Here's how the part is built. I have some questions about the finished solid (model axes, mm). Face numbers are marked on the shaded views. A direction names the side the tool comes from. Round coordinates to 2 decimals unless told otherwise and drop trailing zeros. Loops run counter-clockwise (first coordinate to the right, second up) from the corner with the lowest first, then second, coordinate; pieces in that order, holes last. Notation, with made-up numbers: M 55.25,34.5 L 94.25,34.5 A19 cw 94.25,49.5 Z; hole C 65,82.5 d3. An arc over 180 degrees is marked long. Use a Markdown table: item, result.
```python
from build123d import *

# Parameters (mm, degrees)
F1_DEPTH = 25.4
F0_R     = 19.05
F2_DEPTH = 38.1
F0_R_2   = 6.35
F3_DEPTH = 31.75


with BuildPart() as f1:
    # F0 (on Top) → F1 (new body)
    with BuildSketch(Plane.XY):
        with BuildLine():
            ThreePointArc((256.328097, 0.145331), (242.358097, 12.781672), (256.328097, 25.418012))
            Line((256.328097, 25.418012), (130.598097, 38.054353))
            ThreePointArc((130.598097, 38.054353), (146.895241, 29.82051), (153.458097, 12.781672))
            ThreePointArc((153.458097, 12.781672), (146.895241, -4.257166), (130.598097, -12.491009))
            Line((130.598097, -12.491009), (256.328097, 0.145331))
        make_face()
        with BuildLine():
            ThreePointArc((166.158097, 6.431672), (159.808097, 12.781672), (166.158097, 19.131672))
            Line((166.158097, 19.131672), (216.958097, 19.131672))
            ThreePointArc((216.958097, 19.131672), (223.308097, 12.781672), (216.958097, 6.431672))
            Line((216.958097, 6.431672), (166.158097, 6.431672))
        make_face(mode=Mode.SUBTRACT)
    extrude(amount=F1_DEPTH)

    # F0 (on Top) → F2 (join)
    with BuildSketch(Plane.XY):
        with BuildLine():
            ThreePointArc((153.458097, 12.781672), (146.895241, 29.82051), (130.598097, 38.054353))
            ThreePointArc((130.598097, 38.054353), (102.658097, 12.781672), (130.598097, -12.491009))
            ThreePointArc((130.598097, -12.491009), (146.895241, -4.257166), (153.458097, 12.781672))
        make_face()
        with Locations((128.058097, 12.781672)):
            Circle(F0_R, mode=Mode.SUBTRACT)
    extrude(amount=F2_DEPTH)

    # F0 (on Top) → F3 (join)
    with BuildSketch(Plane.XY):
        with BuildLine():
            ThreePointArc((256.328097, 0.145331), (264.476669, 4.262253), (267.758097, 12.781672))
            ThreePointArc((267.758097, 12.781672), (264.476669, 21.301091), (256.328097, 25.418012))
            ThreePointArc((256.328097, 25.418012), (242.358097, 12.781672), (256.328097, 0.145331))
        make_face()
        with Locations((255.058097, 12.781672)):
            Circle(F0_R_2, mode=Mode.SUBTRACT)
    extrude(amount=F3_DEPTH)


solid = f1.part
```
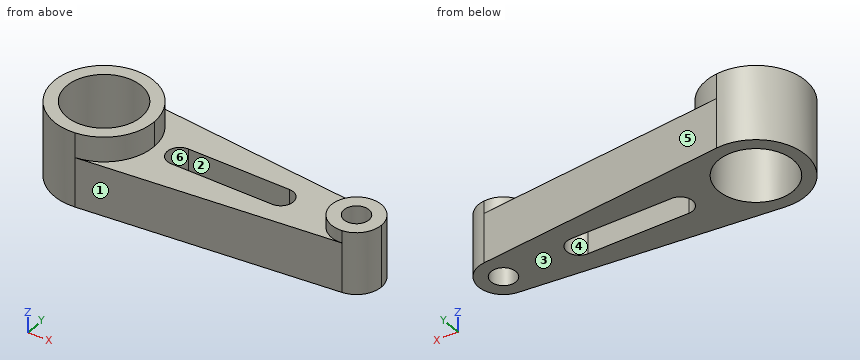
Q1. For the marked faces 1 and 2, which set-ups out of +Z, -Z, +X, -X, +Y, -Y let a thin tool reach every point of the face, with its end or its side?
Return value:
| item | result |
|---|---|
| face 1 | +Z, -Z, +X, -Y |
| face 2 | +Z, -Z |
Q2. Imagine slicing it at D-D, the plane z = 7.5. Please give me the cut outline in (x, y), then the cut area to 3 significant figures.
Return value:
| item | result |
|---|---|
| outline | M 130.6,-12.49 L 256.33,0.15 A12.7 ccw 267.76,12.78 A12.7 ccw 256.33,25.42 L 130.6,38.05 A25.4 ccw long Z; hole C 128.06,12.78 d38.1; hole M 166.16,6.43 L 216.96,6.43 A6.35 ccw 216.96,19.13 L 166.16,19.13 A6.35 ccw Z; hole C 255.06,12.78 d12.7 |
| area | 4,090 mm^2 |
Q3. Imagine slicing it at B-B, the plane x = 194. Please give me the cut outline in (y, z), then the cut area to 3 significant figures.
Return value:
| item | result |
|---|---|
| outline | M -6.12,0 L 6.43,0 L 6.43,25.4 L -6.12,25.4 Z; M 19.13,0 L 31.68,0 L 31.68,25.4 L 19.13,25.4 Z |
| area | 638 mm^2 |
Q4. Will these pins go through, and if not, where does the flat tip stop? P1, Ø8, axis at x = 203, z = 19, coming from the +Y side; P2, Ø3, axis at x = 187, y = -4.5, coming from the +Z side; P3, Ø20.5, axis at x = 191, z = 9.5, coming from the -Y side; P4, Ø10, axis at x = 255.06, y = 12.78, coming from the +Z side.
Return value:
| item | result |
|---|---|
| P1 | stops at y = 31.18 |
| P2 | stops at z = 25.4 |
| P3 | stops at y = -7.45 |
| P4 | passes through |
Q5. We'd pull the mould along X, two halves only. Please class the marked faces 3, 4, 5 and 6: pulls with the +X half, pulls with the -X half, needs draft (parallel to the pull), parting line crosses it, or undercut.
Return value:
| item | result |
|---|---|
| face 3 | needs draft |
| face 4 | undercut |
| face 5 | pulls with the +X half |
| face 6 | undercut |
Q6. I need wall thicknesses on line 1 (X direction, y = 18, z = 26.5); line 2 (X direction, y = 15.5, z = 27); line 3 (X direction, y = 12.5, z = 34). Which ranges of each line are inside material? Lowest first, please. Write a range as from..to.
Return value:
| item | result |
|---|---|
| line 1 | x = 103.2..109.74, 146.38..152.92, 243.48..251.44, 258.68..266.64 |
| line 2 | x = 102.8..109.2, 146.91..153.31, 242.65..249.32, 260.8..267.46 |
| line 3 | x = 102.66..109.01, 147.11..153.46 |
Q7. Imagine slicing it at C-C, the plane y = -2. Please give me the cut outline in (x, z).
Return value:
| item | result |
|---|---|
| outline | M 107.4,0 L 116.04,0 L 116.04,38.1 L 107.4,38.1 Z; M 140.07,0 L 234.98,0 L 234.98,25.4 L 148.71,25.4 L 148.71,38.1 L 140.07,38.1 Z |
Q8. Imagine slicing it at A-A, the plane z = 28.5. Please give me the cut outline in (x, y).
Return value:
| item | result |
|---|---|
| outline | C 128.06,12.78 d50.8; M 256.33,0.15 A12.7 ccw 267.76,12.78 A12.7 ccw long Z; hole C 128.06,12.78 d38.1; hole C 255.06,12.78 d12.7 |
